Here's how the part is built. I have some questions about the finished solid (model axes, mm). Round coordinates to 2 decimals unless told otherwise and drop trailing zeros. Order: outer loops, then holes, each group sorted by start corner. A loop starts at its lowest first (then second) coordinate and runs counter-clockwise, first axis right, second up. Notation, with made-up numbers: M -9,36.5 L 3,36.5 A5 cw 3,41.5 Z; hole C 2,63.5 d1. An arc over 180 degrees is marked long. Write item = value, one per line. Start each with the question number.
Item 1: Please list where these lines run through material, in increasing order: L1, parallel to Z at x = 0, y = 1.8; L2, parallel to X at y = 1.35, z = 0; L3, parallel to Z at x = -8, y = 2.2.
Item 2: We'd pull the mould along X, two halves only. Please class faces 1 (the face through (-1.19, 2.46, 5.37)), 2 (the face through (11.43, 2.54, -20.84)), 3 (the face through (0, 3, -49)): pulls with the +X half, pulls with the -X half, needs draft (parallel to the pull), parting line crosses it, or undercut.
Item 3: I'm going to push flat-ended pins straight in: P1, Ø1.5, axis at x = -11, z = 0, coming from the +Y side; P2, Ø1, axis at y = 0.5, z = -29.5, coming from the +X side; P3, Ø1.5, axis at y = 1, z = -31.5, coming from the -X side. Where does each tip first touch, or does it pass through?
Item 4: I want a section at D-D, the plane y = 3.55. State how many separate pieces and enclosed holes the cut face has, plus the area to 3 significant figures.
Item 5: I want a section at C-C, the plane x = 11. List the corners of the cut face in (y, z) for me, plus the area to 3 significant figures.
Item 6: I want a section at A-A, the plane x = 0. List the corners of the cut face in (y, z) for me.
Item 7: I want a section at B-B, the plane z = -11. List the corners of the cut face in (x, y) for me.
```python
from build123d import *

# Parameters (mm, degrees)
SKETCH1_R                                            = 2.5
SKETCH1_R_2                                          = 5.5
BOSS_EXTRUDE1_DEPTH                                  = 5
SKETCH2_R                                            = 1.25
CUT_EXTRUDE1_DEPTH                                   = 6
CUT_EXTRUDE2_DEPTH                                   = 6
CSK_FOR_M4_HEX_SOCKET_COUNTERSUNK_HEAD_S_D           = 4.5
CSK_FOR_M4_HEX_SOCKET_COUNTERSUNK_HEAD_S_CSINK_D     = 9.18
CSK_FOR_M4_HEX_SOCKET_COUNTERSUNK_HEAD_S_CSINK_ANGLE = 90


with BuildPart() as part:
    # Sketch1 → Boss-Extrude1 (new body)
    with BuildSketch(Plane(origin=(0, 0, 0), x_dir=(1, 0, 0), z_dir=(0, 1, 0))):
        with BuildLine():
            Line((-14, 0), (-14, 40))
            ThreePointArc((-14, 40), (0, 54), (14, 40))
            Line((14, 40), (14, 0))
            ThreePointArc((14, 0), (0, -14), (-14, 0))
        make_face()
        with Locations((0, 40)):
            Circle(SKETCH1_R, mode=Mode.SUBTRACT)
        Circle(SKETCH1_R_2, mode=Mode.SUBTRACT)
    extrude(amount=BOSS_EXTRUDE1_DEPTH)

    # Sketch2 → Cut-Extrude1 (cut, through all)
    with BuildSketch(Plane(origin=(0, 5, 0), x_dir=(1, 0, 0), z_dir=(0, 1, 0))):
        with Locations((0, 11)):
            Circle(SKETCH2_R)
        with Locations((7.778174593, 7.778174593)):
            Circle(SKETCH2_R)
        with Locations((11, 0)):
            Circle(SKETCH2_R)
        with Locations((7.778174593, -7.778174593)):
            Circle(SKETCH2_R)
        with Locations((0, -11)):
            Circle(SKETCH2_R)
        with Locations((-7.778174593, -7.778174593)):
            Circle(SKETCH2_R)
        with Locations((-11, 0)):
            Circle(SKETCH2_R)
        with Locations((-7.778174593, 7.778174593)):
            Circle(SKETCH2_R)
    extrude(amount=-CUT_EXTRUDE1_DEPTH, mode=Mode.SUBTRACT)

    # Sketch3 → Cut-Extrude2 (cut, through all)
    with BuildSketch(Plane(origin=(0, 5, 0), x_dir=(1, 0, 0), z_dir=(0, 1, 0))):
        with BuildLine():
            Line((-14, 40), (-14, 0))
            Line((-14, 0), (-8.932361388, 41.101326486))
            ThreePointArc((-8.932361388, 41.101326486), (0, 49), (8.932361388, 41.101326486))
            Line((8.932361388, 41.101326486), (14, 0))
            Line((14, 0), (14, 40))
            ThreePointArc((14, 40), (0, 54), (-14, 40))
        make_face()
    extrude(amount=-CUT_EXTRUDE2_DEPTH, mode=Mode.SUBTRACT)

    # CSK for M4 Hex Socket Countersunk Head Screw2 (through all)
    with Locations(Plane(origin=(0, 5, 0), x_dir=(1, 0, 0), z_dir=(0, 1, 0))):
        with Locations((0, 40)):
            CounterSinkHole(CSK_FOR_M4_HEX_SOCKET_COUNTERSUNK_HEAD_S_D / 2, CSK_FOR_M4_HEX_SOCKET_COUNTERSUNK_HEAD_S_CSINK_D / 2, counter_sink_angle=CSK_FOR_M4_HEX_SOCKET_COUNTERSUNK_HEAD_S_CSINK_ANGLE)


solid = part.part
```
Filled in:
q1.L1 = -49 to -42.5, -37.5 to -12.25, -9.75 to -5.5, 5.5 to 9.75, 12.25 to 14
q1.L2 = -14 to -12.25, -9.75 to -5.5, 5.5 to 9.75, 12.25 to 14
q1.L3 = -44.12 to -9.01, -6.55 to 6.55, 9.01 to 11.49
q2.face_1 = undercut
q2.face_2 = pulls with the +X half
q2.face_3 = parting line crosses it
q3.P1 = through
q3.P2 = 10.42
q3.P3 = -10.21
q4.separate_pieces = 1
q4.enclosed_holes = 10
q4.area = 1,190 mm^2
q5.outline = M 0,-24.33 L 5,-24.33 L 5,-1.25 L 0,-1.25 Z; M 0,1.25 L 5,1.25 L 5,8.66 L 0,8.66 Z
q5.area = 152 mm^2
q6.outline = M 0,-49 L 5,-49 L 5,-44.59 L 2.91,-42.5 L 0,-42.5 Z; M 0,-37.5 L 2.91,-37.5 L 5,-35.41 L 5,-12.25 L 0,-12.25 Z; M 0,-9.75 L 5,-9.75 L 5,-5.5 L 0,-5.5 Z; M 0,5.5 L 5,5.5 L 5,9.75 L 0,9.75 Z; M 0,12.25 L 5,12.25 L 5,14 L 0,14 Z
q7.outline = M -12.64,0 L -1.25,0 L -1.25,5 L -12.64,5 Z; M 1.25,0 L 12.64,0 L 12.64,5 L 1.25,5 Z
